The listing builds one solid part. Answer for the finished solid, in the listing's coordinates (mm). Face numbers are marked on the shaded views. A direction names the side the tool comes from. Round coordinates to 2 decimals unless told otherwise and drop trailing zeros. Loops run counter-clockwise (first coordinate to the right, second up) from the corner with the lowest first, then second, coordinate; pieces in that order, holes last. Notation, with made-up numbers: (85.25, 66) - (132.25, 66) arc R17 ccw to (132.25, 90) - close; hole circle Ø6 at (17.5, 37.5). An arc over 180 degrees is marked (long way). Write item = value, one per line. Start each with the question number.
1) Section C-C, the plane y = 21 is taken. Determine the outline of the cut face in (x, z).
2) For a pull along Z with two mould halves and no side action, classify the marked faces 4, 5 and 6 as released by +Z, released by -Z, zero draft, split by the parting line, or undercut.
3) A tool of negligible diameter and unlimited length cuts with its end or side. For the marked faces 1, 2 and 3, from which of +Z, -Z, +X, -X, +Y, -Y can it reach the whole face along a straight path? Write none if from no direction.
4) Given pin 1 Ø18.5 at (x, z) = (-37.5, 29) entering from +Y; pin 2 Ø5 at (x, y) = (-57, 13.5) entering from +Z; pin 3 Ø7.5 at (y, z) = (19, 21) entering from +X; pin 4 Ø3 at (x, y) = (-46.5, 16) entering from +Z, each flat-ended and moving along its own axis, determine where each tip first touches the part or whether it passes through.
5) Section D-D, the plane z = 4.5 is taken. Determine the outline of the cut face in (x, y), and give its area (3 significant figures).
6) Straight lines are drawn through the part: line 1 along Z through (x, y) = (-60, 10.5); line 2 along X through (y, z) = (13.75, 14.5); line 3 along Y through (x, z) = (-35.5, 19). For each, find the intervals that lie inside material, in ascending order.
7) Section B-B, the plane y = 18 is taken. Determine the outline of the cut face in (x, z).
8) Section A-A, the plane z = 23.5 is taken. Determine the outline of the cut face in (x, y), and give its area (3 significant figures).
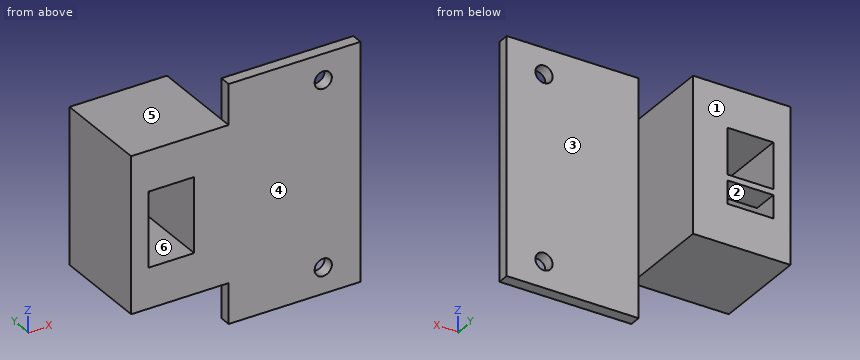
from build123d import *

# Parameters (mm, degrees)
SALIENTE_EXTRUIR1_DEPTH = 41
CROQUIS2_R              = 1.5
CORTAR_EXTRUIR1_DEPTH   = 2
CORTAR_EXTRUIR2_START   = -17
CROQUIS3_W              = 8
CROQUIS3_H              = 13
CROQUIS3_W_2            = 17
CROQUIS3_H_2            = 7
CORTAR_EXTRUIR2_DEPTH   = 17
CROQUIS4_W              = 8
CROQUIS4_H              = 1
SALIENTE_EXTRUIR2_DEPTH = 4.5


with BuildPart() as part:
    # Croquis1 → Saliente-Extruir1 (new body)
    with BuildSketch(Plane.XY):
        Polygon((-65.37305766, 23.186813187), (-48.37305766, 23.186813187), (-48.37305766, 8.186813187), (-25.37305766, 8.186813187), (-25.37305766, 6.186813187), (-65.37305766, 6.186813187), align=None)
    extrude(amount=SALIENTE_EXTRUIR1_DEPTH)

    # Croquis2 → Cortar-Extruir1 (cut)
    with BuildSketch(Plane.XZ.offset(-6.186813187)):
        with Locations((-31.87305766, 36.5)):
            Circle(CROQUIS2_R)
        with Locations((-31.87305766, 4.5)):
            Circle(CROQUIS2_R)
    extrude(amount=-CORTAR_EXTRUIR1_DEPTH, mode=Mode.SUBTRACT)

    # Croquis3 → Cortar-Extruir2 (cut)
    with BuildSketch(Plane.XZ.offset(-6.186813187).offset(CORTAR_EXTRUIR2_START)):
        with Locations((-58.37305766, 20.5)):
            Rectangle(CROQUIS3_W, CROQUIS3_H)
        with Locations((-56.87305766, 37.5)):
            Rectangle(CROQUIS3_W_2, CROQUIS3_H_2)
        with Locations((-56.87305766, 3.5)):
            Rectangle(CROQUIS3_W_2, CROQUIS3_H_2)
    extrude(amount=CORTAR_EXTRUIR2_DEPTH, mode=Mode.SUBTRACT)

    # Croquis4 → Saliente-Extruir2 (add)
    with BuildSketch(Plane(origin=(0, 23.186813187, 0), x_dir=(1, 0, 0), z_dir=(0, 1, 0))):
        with Locations((-58.37305766, -18.5)):
            Rectangle(CROQUIS4_W, CROQUIS4_H)
    extrude(amount=-SALIENTE_EXTRUIR2_DEPTH)


solid = part.part
Geometry check:
q1.outline = (-65.37, 7) - (-48.37, 7) - (-48.37, 34) - (-65.37, 34) - close; hole (-62.37, 14) - (-54.37, 14) - (-54.37, 18) - (-62.37, 18) - close; hole (-62.37, 19) - (-54.37, 19) - (-54.37, 27) - (-62.37, 27) - close
q2.face_4 = zero draft
q2.face_5 = released by +Z
q2.face_6 = undercut
q3.face_1 = +Z, -Z, +X, -X, +Y
q3.face_2 = +Y, -Y
q3.face_3 = +Z, -Z, +X, +Y
q4.pin_1 = 8.19
q4.pin_2 = 34
q4.pin_3 = -48.37
q4.pin_4 = through
q5.outline = (-48.37, 6.19) - (-33.37, 6.19) - (-33.37, 8.19) - (-48.37, 8.19) - close; (-30.37, 6.19) - (-25.37, 6.19) - (-25.37, 8.19) - (-30.37, 8.19) - close
q5.area = 40.0 mm2
q6.line_1 = 7 to 14, 27 to 34
q6.line_2 = -65.37 to -62.37, -54.37 to -48.37
q6.line_3 = 6.19 to 8.19
q7.outline = (-65.37, 7) - (-48.37, 7) - (-48.37, 34) - (-65.37, 34) - close; hole (-62.37, 14) - (-54.37, 14) - (-54.37, 27) - (-62.37, 27) - close
q8.outline = (-65.37, 6.19) - (-62.37, 6.19) - (-62.37, 23.19) - (-65.37, 23.19) - close; (-54.37, 6.19) - (-25.37, 6.19) - (-25.37, 8.19) - (-48.37, 8.19) - (-48.37, 23.19) - (-54.37, 23.19) - close
q8.area = 199 mm2
